Design review of the part built by this model. Coordinates are the model's own, in mm. Coordinates: 2 decimals unless noted, no trailing zeros. Write each loop counter-clockwise with the first axis right and the second up, starting at its lowest first coordinate (ties: lowest second). Pieces come first, ordered by that corner, then holes.
```python
from build123d import *

# Parameters (mm, degrees)
F1_DEPTH = 10


with BuildPart() as f1:
    # F0 (on Front) → F1 (new body)
    with BuildSketch(Plane.XZ):
        Polygon((-11.6566279531, 4.2243999988), (-11.6566279531, 16.7243999988), (-11.6566279531, 29.2243999988), (-36.6566279531, 29.2243999988), (-36.6566279531, 4.2243999988), align=None)
        with BuildLine():
            ThreePointArc((-34.1566279531, 25.4743999988), (-35.0405114295, 27.6082834753), (-32.9066279531, 26.7243999988))
            Line((-32.9066279531, 26.7243999988), (-15.4066279531, 26.7243999988))
            ThreePointArc((-15.4066279531, 26.7243999988), (-14.1566279531, 27.9743999988), (-12.9066279531, 26.7243999988))
            ThreePointArc((-12.9066279531, 26.7243999988), (-13.2727444766, 25.8405165223), (-14.1566279531, 25.4743999988))
            Line((-14.1566279531, 25.4743999988), (-14.1566279531, 16.7243999988))
            Line((-14.1566279531, 16.7243999988), (-14.1566279531, 7.9743999988))
            ThreePointArc((-14.1566279531, 7.9743999988), (-13.2727444766, 7.6082834753), (-12.9066279531, 6.7243999988))
            ThreePointArc((-12.9066279531, 6.7243999988), (-14.1566279531, 5.4743999988), (-15.4066279531, 6.7243999988))
            Line((-15.4066279531, 6.7243999988), (-32.9066279531, 6.7243999988))
            ThreePointArc((-32.9066279531, 6.7243999988), (-35.0405114295, 5.8405165223), (-34.1566279531, 7.9743999988))
            Line((-34.1566279531, 7.9743999988), (-34.1566279531, 16.7243999988))
            Line((-34.1566279531, 16.7243999988), (-34.1566279531, 25.4743999988))
        make_face(mode=Mode.SUBTRACT)
        with BuildLine():
            Line((-14.1566279531, 16.7243999988), (-34.1566279531, 16.7243999988))
            Line((-34.1566279531, 16.7243999988), (-34.1566279531, 7.9743999988))
            ThreePointArc((-34.1566279531, 7.9743999988), (-33.2727444766, 7.6082834753), (-32.9066279531, 6.7243999988))
            Line((-32.9066279531, 6.7243999988), (-15.4066279531, 6.7243999988))
            ThreePointArc((-15.4066279531, 6.7243999988), (-15.0405114295, 7.6082834753), (-14.1566279531, 7.9743999988))
            Line((-14.1566279531, 7.9743999988), (-14.1566279531, 16.7243999988))
        make_face()
        with BuildLine():
            Line((-15.4066279531, 26.7243999988), (-32.9066279531, 26.7243999988))
            ThreePointArc((-32.9066279531, 26.7243999988), (-33.2727444766, 25.8405165223), (-34.1566279531, 25.4743999988))
            Line((-34.1566279531, 25.4743999988), (-34.1566279531, 16.7243999988))
            Line((-34.1566279531, 16.7243999988), (-14.1566279531, 16.7243999988))
            Line((-14.1566279531, 16.7243999988), (-14.1566279531, 25.4743999988))
            ThreePointArc((-14.1566279531, 25.4743999988), (-15.0405114295, 25.8405165223), (-15.4066279531, 26.7243999988))
        make_face()
    extrude(amount=F1_DEPTH)


solid = f1.part
```
(1) Consider section A-A (y = -8.25). Give the boundary of the cut face in (x, z).
(2) Wall thickness on line 1 (Z direction, x = -34.25, y = -5); line 2 (Z direction, x = -33.5, y = -2.5); line 3 (X direction, y = -2.25, z = 25.75): over which ranges is each line inside the solid? List them lowest first.
(3) Insertion check: pin 1 Ø3 at (x, z) = (-34.16, 26.72) entering from -Y; pin 2 Ø1.5 at (x, z) = (-34.16, 6.72) entering from -Y. Each pin has a flat end and moves straight along its axis. Give the tip position at first contact, or say it passes through.
(4) Consider section B-B (z = 6). Give the boundary of the cut face in (x, y).
Results:
1. outline: (-36.66, 4.22) - (-11.66, 4.22) - (-11.66, 29.22) - (-36.66, 29.22) - close; hole circle Ø2.5 at (-34.16, 6.72); hole circle Ø2.5 at (-34.16, 26.72); hole circle Ø2.5 at (-14.16, 6.72); hole circle Ø2.5 at (-14.16, 26.72)
2. line 1: z = 4.22 to 5.48, 7.97 to 25.48, 27.97 to 29.22
2. line 2: z = 4.22 to 5.66, 7.79 to 25.66, 27.79 to 29.22
2. line 3: x = -36.66 to -34.94, -33.37 to -14.94, -13.37 to -11.66
3. pin 1: stops at y = -10
3. pin 2: passes through
4. outline: (-36.66, -10) - (-35.18, -10) - (-35.18, 0) - (-36.66, 0) - close; (-33.14, -10) - (-15.18, -10) - (-15.18, 0) - (-33.14, 0) - close; (-13.14, -10) - (-11.66, -10) - (-11.66, 0) - (-13.14, 0) - close
